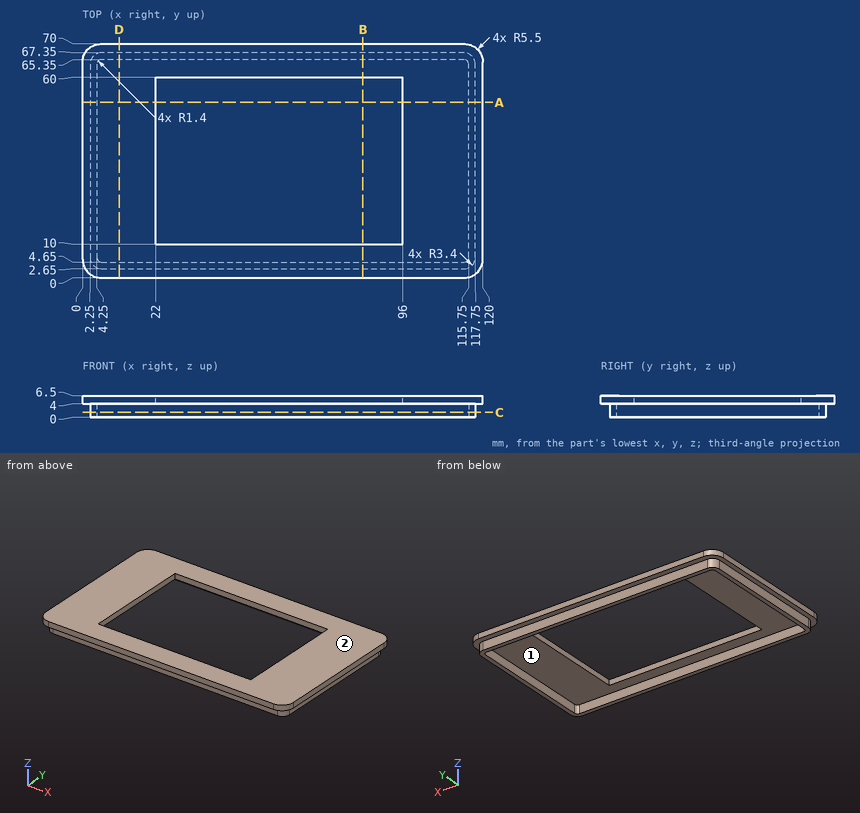
The drawing under review shows one solid part. Ordinate dimensions are in mm from its lowest x, y, z. Coordinates: 2 decimals unless noted, no trailing zeros. Order: outer loops, then holes, each group sorted by start corner. A loop starts at its lowest first (then second) coordinate and runs counter-clockwise, first axis right, second up. Notation, with made-up numbers: (87.25, 7) -> (114.25, 7) arc R5 ccw to (114.25, 14) -> close; hole circle Ø4 at (0, 80.25). An arc over 180 degrees is marked (long way). Answer in a Markdown table with one row per item. Add a question column.
Item 1: Clearance check with flat-ended pins moving along their axes: pin 1 (3 mm diameter, centred on y = 37, z = 5.5, fed in from -X); pin 2 (3 mm diameter, centred on x = 57, z = 1.5, fed in from -Y); pin 3 (10 mm diameter, centred on x = 84.5, y = 51, fed in from +Z); pin 4 (6 mm diameter, centred on x = 18, y = 42.5, fed in from -Z). State where each tip first meets the part, or that it passes through.
Item 2: We need section D-D on x = 11. Write out the cut boundary in (y, z), plus the area to 3 significant figures.
Item 3: To check wall thickness, follow probe 1 along Y at (x, z) = (8, 2.25); probe 2 along X at (y, z) = (8.5, 2); probe 3 along Y at (x, z) = (74.5, 4.25). State the ranges of each line that lie inside material, in increasing order.
Item 4: Mouldability with a two-part tool opening along Y and no side actions: class the marked faces 1 and 2 as +Y half, -Y half, draft (parallel to the pull), parting line (faces both ways), or undercut.
Item 5: We need section A-A on y = 52.5. Write out the cut boundary in (x, z), plus the area to 3 significant figures.
Item 6: We need section C-C on z = 1.5. Write out the cut boundary in (x, y).
Item 7: We need section B-B on x = 84. Write out the cut boundary in (y, z).
Final values:
| question | item | result |
|---|---|---|
| 1 | pin 1 | stops at x = 0 |
| 1 | pin 2 | stops at y = 2.65 |
| 1 | pin 3 | passes through |
| 1 | pin 4 | stops at z = 4 |
| 2 | outline | (0, 4) -> (2.65, 4) -> (2.65, 0) -> (4.65, 0) -> (4.65, 4) -> (65.35, 4) -> (65.35, 0) -> (67.35, 0) -> (67.35, 4) -> (70, 4) -> (70, 6.5) -> (0, 6.5) -> close |
| 2 | area | 191 mm2 |
| 3 | probe 1 | y = 2.65 to 4.65, 65.35 to 67.35 |
| 3 | probe 2 | x = 2.25 to 4.25, 115.75 to 117.75 |
| 3 | probe 3 | y = 0 to 10, 60 to 70 |
| 4 | face 1 | undercut |
| 4 | face 2 | draft |
| 5 | outline | (0, 4) -> (2.25, 4) -> (2.25, 0) -> (4.25, 0) -> (4.25, 4) -> (22, 4) -> (22, 6.5) -> (0, 6.5) -> close; (96, 4) -> (115.75, 4) -> (115.75, 0) -> (117.75, 0) -> (117.75, 4) -> (120, 4) -> (120, 6.5) -> (96, 6.5) -> close |
| 5 | area | 131 mm2 |
| 6 | outline | (2.25, 6.05) arc R3.4 ccw to (5.65, 2.65) -> (114.35, 2.65) arc R3.4 ccw to (117.75, 6.05) -> (117.75, 63.95) arc R3.4 ccw to (114.35, 67.35) -> (5.65, 67.35) arc R3.4 ccw to (2.25, 63.95) -> close; hole (4.25, 6.05) arc R1.4 ccw to (5.65, 4.65) -> (114.35, 4.65) arc R1.4 ccw to (115.75, 6.05) -> (115.75, 63.95) arc R1.4 ccw to (114.35, 65.35) -> (5.65, 65.35) arc R1.4 ccw to (4.25, 63.95) -> close |
| 7 | outline | (0, 4) -> (2.65, 4) -> (2.65, 0) -> (4.65, 0) -> (4.65, 4) -> (10, 4) -> (10, 6.5) -> (0, 6.5) -> close; (60, 4) -> (65.35, 4) -> (65.35, 0) -> (67.35, 0) -> (67.35, 4) -> (70, 4) -> (70, 6.5) -> (60, 6.5) -> close |
